Source: three-view drawing plus pictorial views. Frame: mm from the lowest corner of the part. A direction names the side the tool comes from. Give positions to 0.01 mm unless a question says otherwise; leave off trailing zeros. Order: outer loops, then holes, each group sorted by start corner. A loop starts at its lowest first (then second) coordinate and runs counter-clockwise, first axis right, second up. Notation, with made-up numbers: (-9, -31) - (37, -31) arc R24 ccw to (37, 8) - close; hole circle Ø11 at (30.5, 9). An arc over 180 degrees is marked (long way). Answer in a Markdown table with one row per item. Add a question column.
1. Section query C-C on x = 53. Return loops of the section in (y, z).
2. Ray query, line 1 (X direction, y = 8, z = 63.3); line 2 (X direction, y = 3.25, z = 21.5); line 3 (Z direction, x = 111, y = 8.5). Return the intervals inside material, ascending. Write a range as [from, to].
3. Section query A-A on y = 3.5. Count the separate pieces of the cut face and the enclosed holes in it, and give its area (3 significant figures).
4. Mould query, pull axis Z, two halves, no side actions, for the marked faces 3, 4 and 5. Classes: released by +Z, released by -Z, zero draft, split by the parting line, or undercut.
5. Access query for the marked faces 1 and 2. Directions: +Z, -Z, +X, -X, +Y, -Y. A direction counts if a zero-diameter tool reaches every point of the face in a straight line with its end or side. Return the directions, or none.
6. Section query B-B on z = 13. Return loops of the section in (x, y) (1 decimal).
7. Contact query for flat-ended pins moving along their axis: pin 1 (4 mm diameter, centred on x = 155.96, y = 7.5, fed in from -Z); pin 2 (5 mm diameter, centred on x = 155.96, y = 7.5, fed in from +Z); pin 3 (8 mm diameter, centred on x = 55.5, y = 2, fed in from -Z) (1 decimal); pin 4 (7.5 mm diameter, centred on x = 150, y = 5, fed in from -Z). Output: stop coordinate, or through.
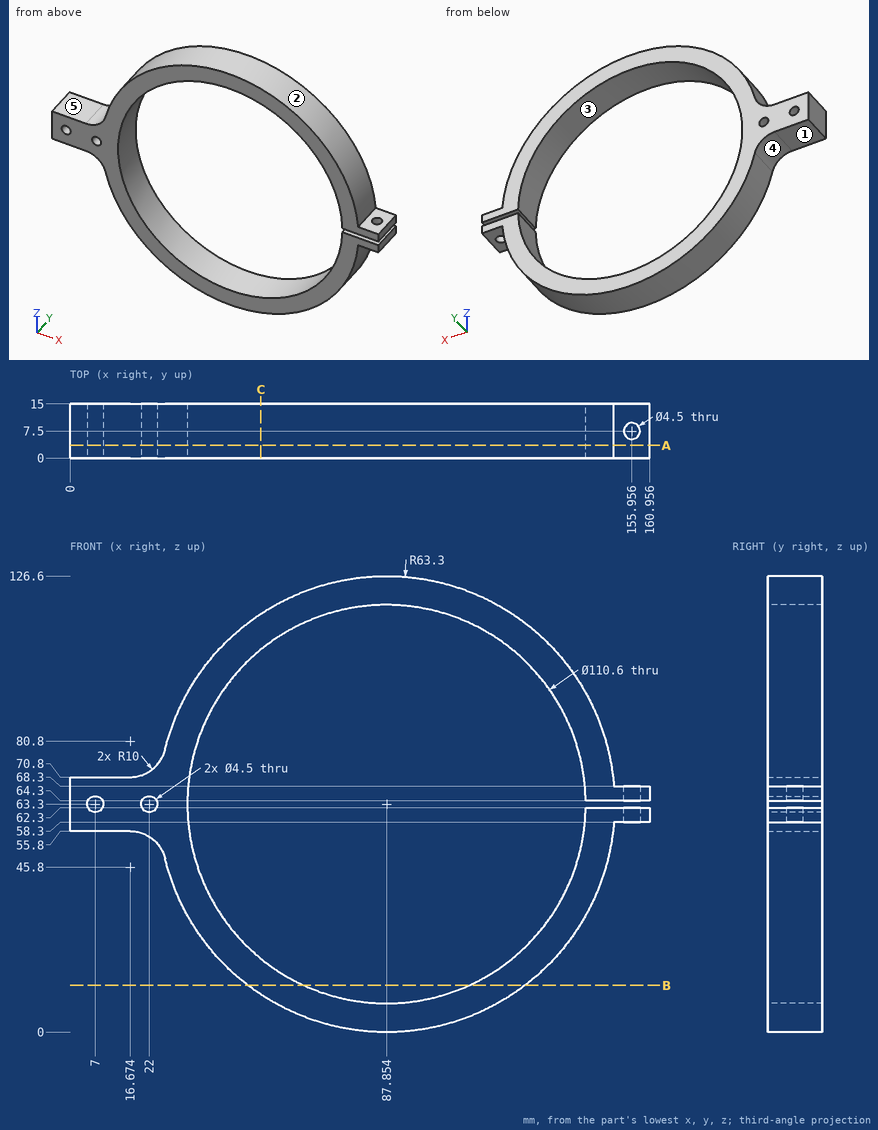
Answer:
| question | item | result |
|---|---|---|
| 1 | outline | (0, 10.46) - (15, 10.46) - (15, 20.37) - (0, 20.37) - close; (0, 106.23) - (15, 106.23) - (15, 116.14) - (0, 116.14) - close |
| 2 | line 1 | x = [0, 4.75], [9.25, 19.75], [24.25, 32.55] |
| 2 | line 2 | x = [40.32, 51.65], [124.06, 135.39] |
| 2 | line 3 | z = [4.38, 13.08], [113.52, 122.22] |
| 3 | separate pieces | 1 |
| 3 | enclosed holes | 2 |
| 3 | area | 3,410 mm² |
| 4 | face 3 | undercut |
| 4 | face 4 | released by -Z |
| 4 | face 5 | released by +Z |
| 5 | face 1 | -Z, -X, +Y, -Y |
| 5 | face 2 | +Z, +Y, -Y |
| 6 | outline | (49.4, 0) - (64.9, 0) - (64.9, 15) - (49.4, 15) - close; (110.8, 0) - (126.3, 0) - (126.3, 15) - (110.8, 15) - close |
| 7 | pin 1 | passes through |
| 7 | pin 2 | stops at z = 68.3 |
| 7 | pin 3 | stops at z = 6.7 |
| 7 | pin 4 | stops at z = 38.87 |
